```python
from build123d import *

# Parameters (mm, degrees)
SKETCH1_R                = 30
SKETCH1_R_2              = 10
BOSS_EXTRUDE1_DEPTH      = 20
BOSS_EXTRUDE1_DEPTH_BACK = 20


with BuildPart() as part:
    # Sketch1 → Boss-Extrude1 (new body, two sides)
    with BuildSketch(Plane(origin=(0, 0, 0), x_dir=(1, 0, 0), z_dir=(0, 1, 0))) as boss_extrude1_sk:
        with BuildLine():
            Line((121.840174455, 98.259716511), (-16.319651091, 36.519433022))
            ThreePointArc((-16.319651091, 36.519433022), (-40, 0), (-16.319651091, -36.519433022))
            Line((-16.319651091, -36.519433022), (121.840174455, -98.259716511))
            ThreePointArc((121.840174455, -98.259716511), (140.88125657, -96.780889591), (150, -80))
            Line((150, -80), (150, 80))
            ThreePointArc((150, 80), (140.88125657, 96.780889591), (121.840174455, 98.259716511))
        make_face()
        Circle(SKETCH1_R, mode=Mode.SUBTRACT)
        with Locations((130, 80)):
            Circle(SKETCH1_R_2, mode=Mode.SUBTRACT)
        with Locations((130, -80)):
            Circle(SKETCH1_R_2, mode=Mode.SUBTRACT)
        with BuildLine():
            Line((60, -5), (120, -5))
            ThreePointArc((120, -5), (125, 0), (120, 5))
            Line((120, 5), (60, 5))
            ThreePointArc((60, 5), (55, 0), (60, -5))
        make_face(mode=Mode.SUBTRACT)
    extrude(amount=BOSS_EXTRUDE1_DEPTH)
    extrude(boss_extrude1_sk.sketch, amount=-BOSS_EXTRUDE1_DEPTH_BACK)


solid = part.part
```
The model under review builds one solid part; all positions refer to its coordinate system, in mm. A direction names the side the tool comes from. Coordinates: 2 decimals unless noted, no trailing zeros. Write each loop counter-clockwise with the first axis right and the second up, starting at its lowest first coordinate (ties: lowest second). Pieces come first, ordered by that corner, then holes.
1) We need section A-A on x = 130. State the section outline as (y, z) points, then the cut area to 3 significant figures.
2) Clearance check with flat-ended pins moving along their axes: pin 1 Ø18 at (x, z) = (130, 80) entering from -Y; pin 2 Ø10 at (x, y) = (102, -13.5) entering from +Z; pin 3 Ø8 at (y, z) = (-1, 54) entering from -X; pin 4 Ø6 at (x, y) = (50, -6) entering from +Z. State where each tip first meets the part, or that it passes through.
3) We need section D-D on x = 71.5. State the section outline as (y, z) points, then the cut area to 3 significant figures.
4) Machinability: for faces 1 (the face through (75, -20, 21)), 2 (the face through (90, 0, 5)), which of the approach directions +Z, -Z, +X, -X, +Y, -Y give a long, thin tool a straight path to every point of the face, cutting with its end or side? Answer none if there is none.
5) To check wall thickness, follow probe 1 along Z at (x, y) = (130, 2); probe 2 along X at (y, z) = (-7, 0); probe 3 along Z at (x, y) = (95, 17). State the ranges of each line that lie inside material, in increasing order.
6) The part is to be moulded in two halves that separate along Z. For faces 3 (the face through (128.698, -0.28, 70.085)), 4 (the face through (140.65, 0.28, 96.93)), 5 (the face through (141.11, 0.28, -96.63)), say which applies: pulls with the +Z half, pulls with the -Z half, needs draft (parallel to the pull), parting line crosses it, or undercut.
7) We need section B-B on z = 0. State the section outline as (x, y) points.
8) We need section C-C on y = -17. State the section outline as (x, z) points.
Answer list:
1. outline: (-20, -100) - (20, -100) - (20, -90) - (-20, -90) - close; (-20, -70) - (20, -70) - (20, 70) - (-20, 70) - close; (-20, 90) - (20, 90) - (20, 100) - (-20, 100) - close
1. area: 6,400 mm2
2. pin 1: passes through
2. pin 2: stops at z = 91.63
2. pin 3: stops at x = 13.85
2. pin 4: stops at z = 67.5
3. outline: (-20, -75.76) - (20, -75.76) - (20, -5) - (-20, -5) - close; (-20, 5) - (20, 5) - (20, 75.76) - (-20, 75.76) - close
3. area: 5,660 mm2
4. face 1: +Z, -Z, +X, -X, -Y
4. face 2: +Y, -Y
5. probe 1: z = -100 to -90, -70 to 70, 90 to 100
5. probe 2: x = -40 to -30, 30 to 55, 125 to 150
5. probe 3: z = -86.27 to -5, 5 to 86.27
6. face 3: undercut
6. face 4: pulls with the +Z half
6. face 5: pulls with the -Z half
7. outline: (-40, -20) - (-30, -20) - (-30, 20) - (-40, 20) - close; (30, -20) - (55, -20) - (55, 20) - (30, 20) - close; (125, -20) - (150, -20) - (150, 20) - (125, 20) - close
8. outline: (-16.32, -36.52) - (121.84, -98.26) arc R20 ccw to (150, -80) - (150, 80) arc R20 ccw to (121.84, 98.26) - (-16.32, 36.52) arc R40 ccw to start; hole circle Ø60 at (0, 0); hole (60, -5) - (120, -5) arc R5 ccw to (120, 5) - (60, 5) arc R5 ccw to start; hole circle Ø20 at (130, -80); hole circle Ø20 at (130, 80)
